from build123d import *

# Parameters (mm, degrees)
F0_R     = 23.208825
F1_DEPTH = 25.4
F2_R     = 5.08
F3_R     = 48.138061
F4_DEPTH = 69.56518


with BuildPart() as f1:
    # F0 (on Top) → F1 (new body)
    with BuildSketch(Plane.XY):
        Circle(F0_R)
    extrude(amount=F1_DEPTH)

    # F2
    f2_edges = [f1.edges().sort_by_distance(p)[0] for p in [
        (-23.208825, 0, 0),
        (-23.208825, 0, 25.4),
    ]]
    fillet(f2_edges, radius=F2_R)

    # F3 (on face) → F4 (join)
    with BuildSketch(Plane(origin=(0, 0, 0), x_dir=(1, 0, 0), z_dir=(0, 0, -1))):
        Circle(F3_R)
    extrude(amount=F4_DEPTH)


solid = f1.part
Input: part model. Units: mm. Frame: model coordinates. A direction names the side the tool comes from. Give positions to 0.01 mm unless a question says otherwise; leave off trailing zeros. Order: outer loops, then holes, each group sorted by start corner. A loop starts at its lowest first (then second) coordinate and runs counter-clockwise, first axis right, second up. Notation, with made-up numbers: (20, 5) -> (68, 5) arc R19 cw to (68, 9) -> close; hole circle Ø1 at (0.25, -2). An arc over 180 degrees is marked (long way). Use one line per item in the form item = value.
1) Section D-D, the plane z = 12. Return loops of the section in (x, y).
Response values:
outline = circle Ø46.42 at (0, 0)
2) First-contact query: pin 1 Ø2 at (x, z) = (32.5, -13) entering from -Y; pin 2 Ø2 at (x, z) = (-20, -17) entering from +Y; pin 3 Ø1 at (y, z) = (34.5, -49) entering from -X. Flat tips, straight axial feed; report the tip coordinate or a pass-through.
Response values:
pin_1 = -36.4
pin_2 = 44.23
pin_3 = -34.08
3) Section C-C, the plane z = -33. Return loops of the section in (x, y), and give its area (3 significant figures).
Response values:
outline = circle Ø96.28 at (0, 0)
area = 7,280 mm^2
4) Reachability of faces 1 (the cylindrical face through (-23.186, 1.02, 12.593)), 2 (the cylindrical face through (25.88, -40.59, -34.3)) from +Z, -Z, +X, -X, +Y, -Y: full face, straight path, thin tool, end or side. Return the list, or none.
Response values:
face_1 = +Z
face_2 = +Z, -Z
5) Line query: probe 1 along Z at (x, y) = (-1.5, -37.5); probe 2 along Y at (x, z) = (18.5, 12.5); probe 3 along X at (y, z) = (31.5, -52.5). Output: solid intervals per line, ascending.
Response values:
probe_1 = -69.57 to 0
probe_2 = -14.01 to 14.01
probe_3 = -36.4 to 36.4
6) Section A-A, the plane x = 0. Return loops of the section in (y, z), and give its area (3 significant figures).
Response values:
outline = (-48.14, -69.57) -> (48.14, -69.57) -> (48.14, 0) -> (18.13, 0) arc R5.08 ccw to (23.21, 5.08) -> (23.21, 20.32) arc R5.08 ccw to (18.13, 25.4) -> (-18.13, 25.4) arc R5.08 ccw to (-23.21, 20.32) -> (-23.21, 5.08) arc R5.08 ccw to (-18.13, 0) -> (-48.14, 0) -> close
area = 7,850 mm^2
